Geometry check sheet. Reference: the model listing, model coordinates, mm. Face numbers are marked on the shaded views. A direction names the side the tool comes from. Round coordinates to 2 decimals unless told otherwise and drop trailing zeros. Order: outer loops, then holes, each group sorted by start corner. A loop starts at its lowest first (then second) coordinate and runs counter-clockwise, first axis right, second up.
(1) Sectioned sample at A-A (x = 2.75). Record the boundary of the cut face in (y, z).
(2) Set-up check for the marked faces 1 and 2: record each of +Z, -Z, +X, -X, +Y, -Y from which the full face is reachable in a straight line by a thin tool's end or side.
(3) Sectioned sample at B-B (z = 2.25). Record the boundary of the cut face in (x, y), plus the area to 3 significant figures.
(4) Sectioned sample at D-D (x = 9.75). Record the boundary of the cut face in (y, z), plus the area to 3 significant figures.
(5) Go/stop test with a flat-tipped pin: pin 1 (1 mm diameter, centred on x = 13, z = 7, fed in from -Y). Record where the tip stops, or that it passes through.
(6) Material ranges on line 1 along Y through (x, z) = (23.25, 2.5); line 2 along X through (y, z) = (-2.5, 4.5); line 3 along X through (y, z) = (8, 8.5), recorded low to high.
from build123d import *

# Parameters (mm, degrees)
RESSALTO_EXTRUS_O1_DEPTH = 10
ESBO_O2_R                = 3.5
RESSALTO_EXTRUS_O2_DEPTH = 4


with BuildPart() as part:
    # Esboço1 → Ressalto-extrusão1 (new body)
    with BuildSketch(Plane(origin=(0, 0, 0), x_dir=(1, 0, 0), z_dir=(0, 1, 0))):
        with BuildLine():
            Line((0, 0), (20, 0))
            ThreePointArc((20, 0), (24.566666667, -4.566666667), (20, -9.133333333))
            Line((20, -9.133333333), (0, -9.133333333))
            ThreePointArc((0, -9.133333333), (-4.566666667, -4.566666667), (0, 0))
        make_face()
    extrude(amount=RESSALTO_EXTRUS_O1_DEPTH)

    # Esboço2 → Ressalto-extrusão2 (add)
    with BuildSketch(Plane(origin=(0, 0, 0), x_dir=(1, 0, 0), z_dir=(0, 1, 0))):
        with Locations(Location((0, -4.566666667, 0), (0, 0, 270))):
            Circle(ESBO_O2_R)
    extrude(amount=-RESSALTO_EXTRUS_O2_DEPTH)


solid = part.part
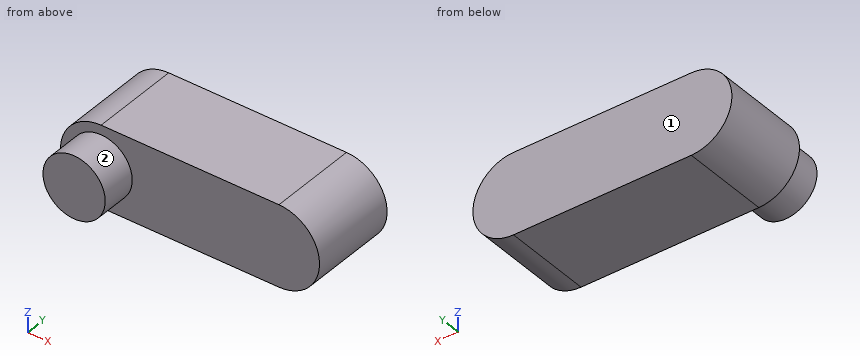
Answer below:
1. outline: (-4, 2.4) - (0, 2.4) - (0, 0) - (10, 0) - (10, 9.13) - (0, 9.13) - (0, 6.73) - (-4, 6.73) - close
2. face 1: +Z, -Z, +X, -X, +Y
2. face 2: -Y
3. outline: (-3.94, 0) - (-2.62, 0) - (-2.62, -4) - (2.62, -4) - (2.62, 0) - (23.94, 0) - (23.94, 10) - (-3.94, 10) - close
3. area: 300 mm2
4. outline: (0, 0) - (10, 0) - (10, 9.13) - (0, 9.13) - close
4. area: 91.3 mm2
5. pin 1: stops at y = 0
6. line 1: y = 0 to 10
6. line 2: x = -3.5 to 3.5
6. line 3: x = -2.32 to 22.32
